Geometry: final body of the model. Coordinates: model frame, mm. Face numbers are marked on the shaded views. Give positions to 0.01 mm unless a question says otherwise; leave off trailing zeros. Write each loop counter-clockwise with the first axis right and the second up, starting at its lowest first coordinate (ties: lowest second). Pieces come first, ordered by that corner, then holes. Notation, with made-up numbers: (79, 14.25) -> (108, 14.25) arc R22 ccw to (108, 40.25) -> close; hole circle Ø6 at (-28, -37.5). An arc over 180 degrees is marked (long way). Answer as a JSON object with one key per item and string values.
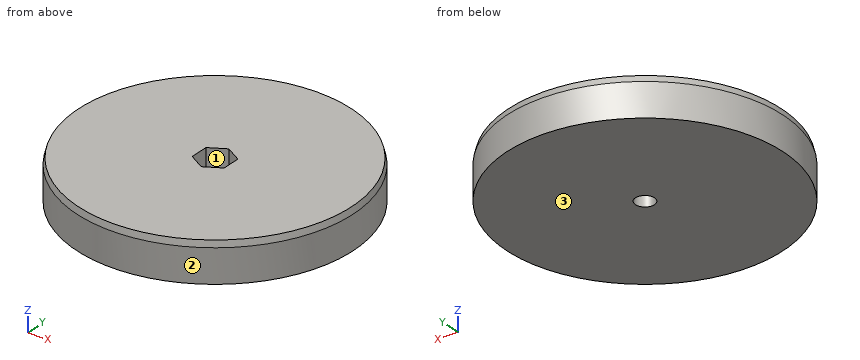
from build123d import *

# Parameters (mm, degrees)
SKETCH001_R       = 3.05
POCKET_DEPTH      = 0.001
POCKET_DEPTH_BACK = -12.701
POCKET001_DEPTH   = 6


with BuildPart() as part:
    # Sketch → Revolution (revolve)
    with BuildSketch(Plane.YZ):
        Polygon((0, 12.7), (43.5, 12.7), (44, 10.7), (44, 0), (0, 0), align=None)
    revolve(axis=Axis((0, 0, 0), (0, 0, 1)))

    # Sketch001 → Pocket (cut, two sides)
    with BuildSketch(Plane.XY) as pocket_sk:
        Circle(SKETCH001_R)
    extrude(amount=-POCKET_DEPTH, mode=Mode.SUBTRACT)
    extrude(pocket_sk.sketch, amount=-POCKET_DEPTH_BACK, mode=Mode.SUBTRACT)

    # Sketch002 → Pocket001 (cut)
    with BuildSketch(Plane.XY.offset(12.7)):
        Polygon((0, 5.888973), (-5.1, 2.944486), (-5.1, -2.944486), (0, -5.888973), (5.1, -2.944486), (5.1, 2.944486), align=None)
    extrude(amount=-POCKET001_DEPTH, mode=Mode.SUBTRACT)


solid = part.part
Q1. Cut plane A-A (y = 0). Return the cut outline in (x, z).
Values:
{"outline": "(-44, 0) -> (-3.05, 0) -> (-3.05, 6.7) -> (-5.1, 6.7) -> (-5.1, 12.7) -> (-43.5, 12.7) -> (-44, 10.7) -> close; (3.05, 0) -> (44, 0) -> (44, 10.7) -> (43.5, 12.7) -> (5.1, 12.7) -> (5.1, 6.7) -> (3.05, 6.7) -> close"}
Q2. Material intervals for L1, parallel to X at y = 0, z = 5; L2, parallel to Y at x = -4, z = 10.25, sorted ascending. Write a range as from..to.
Values:
{"L1": "-44..-3.05, 3.05..44", "L2": "-43.82..-3.58, 3.58..43.82"}
Q3. First-contact query: P1, Ø1.5, axis at y = -23, z = 2, coming from the -X side; P2, Ø3.5, axis at x = 0, y = 0, coming from the +Z side; P3, Ø3, axis at y = -18.5, z = 5, coming from the -X side; P4, Ø3, axis at x = 13, z = 7.5, coming from the -Y side. Flat tips, straight axial feed; report the tip coordinate or a pass-through.
Values:
{"P1": "x = -37.96", "P2": "through", "P3": "x = -40.58", "P4": "y = -42.47"}
Q4. Cut plane B-B (z = 3.25). Return the cut outline in (x, y).
Values:
{"outline": "circle Ø88 at (0, 0); hole circle Ø6.1 at (0, 0)"}
Q5. Mould query, pull axis X, two halves, no side actions, for the marked faces 1, 2 and 3. Classes: pulls with the +X half, pulls with the -X half, needs draft (parallel to the pull), parting line crosses it, or undercut.
Values:
{"face 1": "undercut", "face 2": "parting line crosses it", "face 3": "needs draft"}
